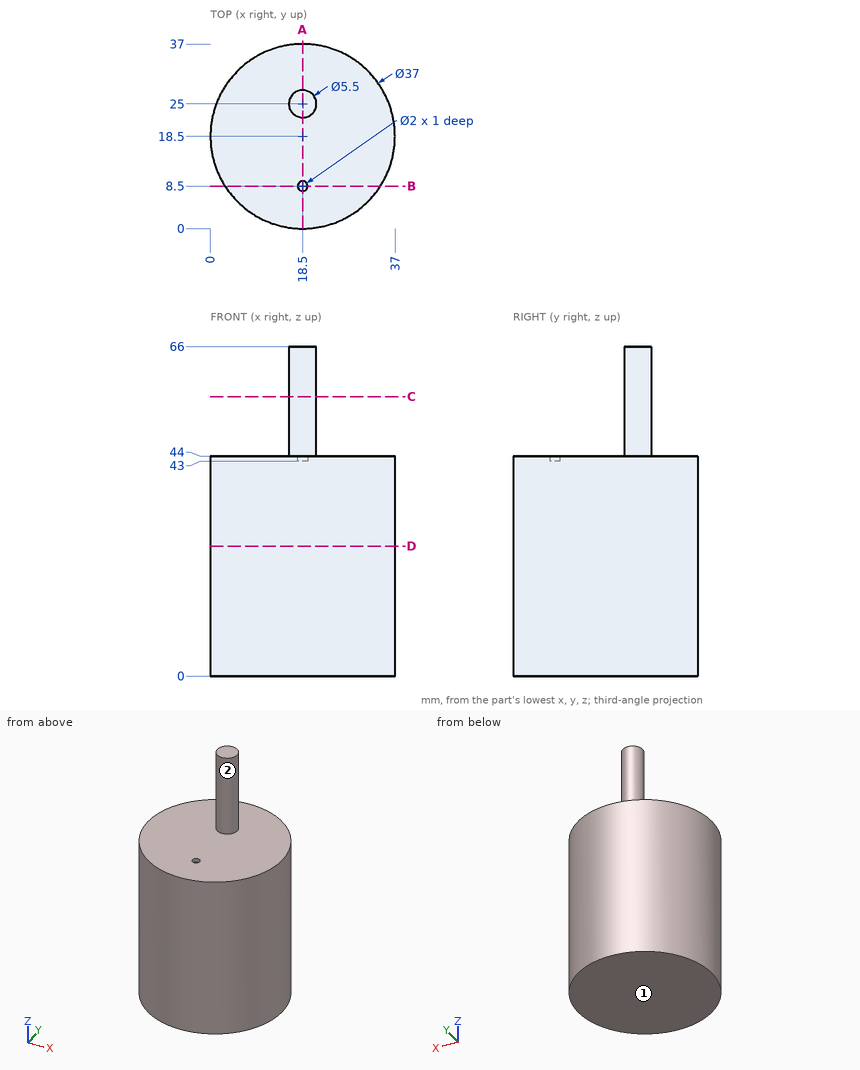
Design review of the part shown in the three views and the two pictorial views. Dimensions are in mm from the part's minimum x, y and z. A direction names the side the tool comes from. Round coordinates to 2 decimals unless told otherwise and drop trailing zeros. Write each loop counter-clockwise with the first axis right and the second up, starting at its lowest first coordinate (ties: lowest second). Pieces come first, ordered by that corner, then holes. Notation, with made-up numbers: (29, 35.5) - (41, 35.5) arc R10 ccw to (41, 52.5) - close; hole circle Ø8 at (-22, -39.75). An arc over 180 degrees is marked (long way). Write item = value, one per line. Start each with the question number.
1. Consider section A-A on x = 18.5. State the section outline as (y, z) points.
2. Consider section C-C on z = 56. State the section outline as (x, y) points, plus the area to 3 significant figures.
3. For pin 1 Ø10 at (y, z) = (32, 25.5) entering from +X; pin 2 Ø12 at (y, z) = (25, 11) entering from +X; pin 3 Ø4 at (x, z) = (30, 19.5) entering from -Y, all flat-tipped, find the tip position at first contact; note any pin that passes through.
4. Consider section B-B on y = 8.5. State the section outline as (x, z) points, plus the area to 3 significant figures.
5. For the marked faces 1 and 2, list the 3-axis set-ups (+Z, -Z, +X, -X, +Y, -Y) from which the entire face can be reached by the end or side of a thin tool; tool diameter is ignored.
6. Consider section D-D on z = 26. State the section outline as (x, y) points, plus the area to 3 significant figures.
7. Wall thickness on L1, parallel to Z at x = 29.5, y = 8.5; L2, parallel to Y at x = 18.5, z = 43.5; L3, parallel to X at y = 3.5, z = 27: over which ranges is each line inside the solid? List them lowest first.
Evaluation:
q1.outline = (0, 0) - (37, 0) - (37, 44) - (27.75, 44) - (27.75, 66) - (22.25, 66) - (22.25, 44) - (9.5, 44) - (9.5, 43) - (7.5, 43) - (7.5, 44) - (0, 44) - close
q2.outline = circle Ø5.5 at (18.5, 25)
q2.area = 23.8 mm2
q3.pin_1 = 34.93
q3.pin_2 = 36.99
q3.pin_3 = 2.63
q4.outline = (2.94, 0) - (34.06, 0) - (34.06, 44) - (19.5, 44) - (19.5, 43) - (17.5, 43) - (17.5, 44) - (2.94, 44) - close
q4.area = 1,370 mm2
q5.face_1 = -Z, +X, -X, +Y, -Y
q5.face_2 = +Z
q6.outline = circle Ø37 at (18.5, 18.5)
q6.area = 1,080 mm2
q7.L1 = 0 to 44
q7.L2 = 0 to 7.5, 9.5 to 37
q7.L3 = 7.67 to 29.33
